Geometry check sheet. Reference: the model listing, model coordinates, mm. A direction names the side the tool comes from. Give positions to 0.01 mm unless a question says otherwise; leave off trailing zeros. Order: outer loops, then holes, each group sorted by start corner. A loop starts at its lowest first (then second) coordinate and runs counter-clockwise, first axis right, second up.
```python
from build123d import *

# Parameters (mm, degrees)
SKETCH_1_W      = 16
SKETCH_1_H      = 30
EXTRUDE_1_DEPTH = 18
EXTRUDE_2_DEPTH = 5


with BuildPart() as part:
    # Эскиз1 → Бобышка-Вытянуть1 (new body)
    with BuildSketch(Plane(origin=(0, 0, 0), x_dir=(1, 0, 0), z_dir=(0, 1, 0))):
        with Locations((8, 15)):
            Rectangle(SKETCH_1_W, SKETCH_1_H)
    extrude(amount=EXTRUDE_1_DEPTH)

    # Эскиз2 → Бобышка-Вытянуть2 (add)
    with BuildSketch(Plane.XZ):
        Polygon((7.25, -15), (7.25, 0), (8.75, 0), (8.75, -15), (8.75, -30), (7.25, -30), align=None)
    extrude(amount=EXTRUDE_2_DEPTH)


solid = part.part
```
Q1. Gauge pin test, flat ends, axial feed: P1, Ø6, axis at x = 12, z = -22.5, coming from the -Y side; P2, Ø4, axis at y = -2.5, z = -5.5, coming from the -X side; P3, Ø2.5, axis at y = -1.5, z = -13.5, coming from the +X side. Record the tip position at first contact, or that the pin passes through.
Q2. Cross-section at C-C, the plane x = 10.75. Record the boundary of the cut face in (y, z), and give its area (3 significant figures).
Q3. Thickness scan on L1, parallel to Y at x = 10.5, z = -2.5; L2, parallel to X at y = -0.5, z = -4.75. Record the ranges inside material, lowest first.
Q4. Cross-section at B-B, the plane y = -2. Record the boundary of the cut face in (x, z).
Q5. Access from +Z, -Z, +X, -X, +Y, -Y to the whole of each face (thin tool, end or side, straight path). Record for faces 1 (the face through (0, 9, -15)), 2 (the face through (12, 0, -15)), 3 (the face through (4, 0, -15)).
Q6. Cross-section at A-A, the plane z = -27.75. Record the boundary of the cut face in (x, y), and give its area (4 significant figures).
Answers follow:
1. P1: stops at y = 0
1. P2: stops at x = 7.25
1. P3: stops at x = 8.75
2. outline: (0, -30) - (18, -30) - (18, 0) - (0, 0) - close
2. area: 540 mm2
3. L1: y = 0 to 18
3. L2: x = 7.25 to 8.75
4. outline: (7.25, -30) - (8.75, -30) - (8.75, 0) - (7.25, 0) - close
5. face 1: +Z, -Z, -X, +Y, -Y
5. face 2: +Z, -Z, +X, -Y
5. face 3: +Z, -Z, -X, -Y
6. outline: (0, 0) - (7.25, 0) - (7.25, -5) - (8.75, -5) - (8.75, 0) - (16, 0) - (16, 18) - (0, 18) - close
6. area: 295.5 mm2
